Geometry check sheet. Reference: the model listing, model coordinates, mm. A direction names the side the tool comes from. Coordinates: 2 decimals unless noted, no trailing zeros. Write each loop counter-clockwise with the first axis right and the second up, starting at its lowest first coordinate (ties: lowest second). Pieces come first, ordered by that corner, then holes. Notation, with made-up numbers: (-16, -36) -> (30, -36) arc R24 cw to (30, -5) -> close; hole circle Ø9 at (79.5, 78.5). An arc over 180 degrees is marked (long way). Answer in a Markdown table with one row per item. Add a question column.
Q1. Release check for a two-part mould opening along X. For faces 3 (the face through (7, 8.922, 5)), 4 (the face through (11.127, -1.846, -7.249)), 5 (the face through (3.05, 2.4, -6.2)) record: pulls with the +X half, pulls with the -X half, needs draft (parallel to the pull), parting line crosses it, or undercut.
Q2. Tool access check on faces 1 (the face through (-3, -3.778, -5)), 2 (the face through (-7.4, 4.4, -2.9)). Record the directions out of +Z, -Z, +X, -X, +Y, -Y that give a thin tool (end or side, any length) a straight path to the whole face; none if there is none.
Q3. Section check D-D, the plane y = -1.75. Record the boundary of the cut face in (x, z), and give its area (3 significant figures).
Q4. Section check A-A, the plane z = 0. Record the boundary of the cut face in (x, y), and give its area (3 significant figures).
Q5. Thickness scan on line 1 (X direction, y = 4, z = 5); line 2 (X direction, y = 6.75, z = -2.5); line 3 (Y direction, x = 11.5, z = -2.75). Record the ranges inside material, lowest first.
Q6. Section check C-C, the plane x = -7.5. Record the boundary of the cut face in (y, z).
Q7. Section check B-B, the plane y = 4.5. Record the boundary of the cut face in (x, z) (3 decimals), and give its area (3 significant figures).
Q8. Gauge pin test, flat ends, axial feed: P1, Ø2, axis at x = 2, y = 3, coming from the +Z side (3 decimals); P2, Ø6, axis at x = -5.5, y = 7, coming from the +Z side; P3, Ø5, axis at y = -1, z = 9, coming from the +X side; P4, Ø2, axis at x = -2.5, z = -2, coming from the -Y side. Record the tip position at first contact, or that the pin passes through.
Autodesk Inventor part; units mm, degrees
ref_plane "YZ Plane" through (0, 0, 0) normal (1, 0, 0) x (0, 1, 0)
ref_plane "XZ Plane" through (0, 0, 0) normal (0, 1, 0) x (-1, 0, 0)
ref_plane "XY Plane" through (0, 0, 0) normal (0, 0, 1) x (1, 0, 0)
sketch "Sketch1" plane through (0, 0, 0) normal (0, 0, 1) x (1, 0, 0)
  line L0 (-4.6769, 8.9222) -> (-7.8519, 8.9222)
  line L1 (-7.8519, 8.9222) -> (-7.8519, 0.0322)
  line L2 (-7.8519, -3.7778) -> (-4.6769, -3.7778)
  line L3 (1.6731, -3.7778) -> (1.6731, 8.9222)
  line L4 (-4.6769, -3.7778) -> (-10.2395, -3.7778)
  line L5 (-10.2395, -3.7778) -> (-10.2395, 0.0322)
  line L6 (-10.2395, 0.0322) -> (-7.8519, 0.0322)
  line L7 (1.6731, 3.6296) -> (1.6731, -3.7778)
  line L8 (-4.6769, -3.7778) -> (-4.6769, 8.9222)
  point P0 (0, 0)
  dimension "d0" = 12.7
  dimension "d1" = 11.9126
  dimension "d2" = 9.525
  dimension "d3" = 6.35
  dimension "d4" = 3.81
revolve "Revolution1" add sketch "Sketch1" angle 360 about axis through (1.6731, -3.7778, 0) along (0, 1, 0)
chamfer "Chamfer1" distance 0.635 angle 45 1 edges at (8.0231, 8.9222, 0)
fillet "Fillet1" radius 0.127 1 edges at (8.0231, -3.7778, 0)
properties part number "Ratchet Bushing 1764"
Calculated:
| question | item | result |
|---|---|---|
| 1 | face 3 | needs draft |
| 1 | face 4 | parting line crosses it |
| 1 | face 5 | undercut |
| 2 | face 1 | +Z, -Z, +X, -X, -Y |
| 2 | face 2 | +Y |
| 3 | outline | circle Ø23.83 at (1.67, 0); hole circle Ø12.7 at (1.67, 0) |
| 3 | area | 319 mm² |
| 4 | outline | (-10.24, -3.78) -> (-4.8, -3.78) arc R0.13 ccw to (-4.68, -3.65) -> (-4.68, 8.29) -> (-5.31, 8.92) -> (-7.85, 8.92) -> (-7.85, 0.03) -> (-10.24, 0.03) -> close; (8.02, -3.65) arc R0.13 ccw to (8.15, -3.78) -> (13.59, -3.78) -> (13.59, 0.03) -> (11.2, 0.03) -> (11.2, 8.92) -> (8.66, 8.92) -> (8.02, 8.29) -> close |
| 4 | area | 98.4 mm² |
| 5 | line 1 | x = -6.43 to -2.24, 5.59 to 9.78 |
| 5 | line 2 | x = -7.52 to -4.16, 7.51 to 10.86 |
| 5 | line 3 | y = -3.78 to 0.03 |
| 6 | outline | (-3.78, -7.6) -> (0.03, -7.6) -> (0.03, -2.57) -> (8.92, -2.57) -> (8.92, 2.57) -> (0.03, 2.57) -> (0.03, 7.6) -> (-3.78, 7.6) -> close |
| 7 | outline | circle Ø19.05 at (1.673, 0); hole circle Ø12.7 at (1.673, 0) |
| 7 | area | 158 mm² |
| 8 | P1 | stops at z = 9.525 |
| 8 | P2 | stops at z = 8.56 |
| 8 | P3 | stops at x = 11.66 |
| 8 | P4 | passes through |
